Source: CAD feature listing. Evaluate the final solid. Frame: model axes, mm. Face numbers are marked on the shaded views. A direction names the side the tool comes from. Give positions to 0.01 mm unless a question says otherwise; leave off trailing zeros. Loops run counter-clockwise (first coordinate to the right, second up) from the corner with the lowest first, then second, coordinate; pieces in that order, holes last. Notation, with made-up numbers: (54.5, -34) -> (93.5, -34) arc R16 cw to (93.5, -23) -> close; hole circle Ø8 at (5.5, -2). An arc over 180 degrees is marked (long way). Return JSON: item names as keys, results as strings. Group by question number.
```python
from build123d import *

# Parameters (mm, degrees)
SKETCH2_W            = 230
SKETCH2_H            = 40
BOSS_EXTRUDE1_DEPTH  = 80
SKETCH3_W            = 200.4
SKETCH3_H            = 10
CUT_EXTRUDE1_DEPTH   = 30
SKETCH6_R            = 25
BOSS_EXTRUDE3_DEPTH  = 50
SKETCH7_R            = 12.5
CUT_EXTRUDE2_DEPTH   = 50
SKETCH8_R            = 26.5
CUT_EXTRUDE3_DEPTH   = 25
CUT_EXTRUDE4_START   = 40
SKETCH11_R           = 26.5
CUT_EXTRUDE4_DEPTH   = 40
SKETCH14_W           = 12.614661349
SKETCH14_H           = 40
CUT_EXTRUDE6_DEPTH   = 50
FILLET3_R            = 20
FILLET3_OF_MIRROR5_R = 20
FILLET3_OF_MIRROR8_R = 20
SKETCH15_R           = 27.771194789
CUT_EXTRUDE7_DEPTH   = 5
SKETCH21_R           = 27.635802496
CUT_EXTRUDE8_DEPTH   = 5


with BuildPart() as part:
    # Sketch2 → Boss-Extrude1 (new body)
    with BuildSketch(Plane.XY):
        with Locations((115, 20)):
            Rectangle(SKETCH2_W, SKETCH2_H)
    extrude(amount=BOSS_EXTRUDE1_DEPTH)

    # Sketch3 → Cut-Extrude1 (cut)
    with BuildSketch(Plane.XY.offset(80)):
        with Locations((115, 20)):
            Rectangle(SKETCH3_W, SKETCH3_H)
    extrude(amount=-CUT_EXTRUDE1_DEPTH, mode=Mode.SUBTRACT)

    # Sketch6 → Boss-Extrude3 (add)
    with BuildSketch(Plane(origin=(140, 0, 0), x_dir=(0, 0, -1), z_dir=(1, 0, 0))):
        with Locations((10, 20)):
            Circle(SKETCH6_R)
    boss_extrude3 = extrude(amount=BOSS_EXTRUDE3_DEPTH)

    # Sketch7 → Cut-Extrude2 (cut)
    with BuildSketch(Plane.ZY.offset(-140)):
        with Locations(Location((-10, 20, 0), (0, 0, 36.869897646))):
            Circle(SKETCH7_R)
    cut_extrude2 = extrude(amount=-CUT_EXTRUDE2_DEPTH, mode=Mode.SUBTRACT)

    # Sketch8 → Cut-Extrude3 (cut)
    with BuildSketch(Plane.ZY.offset(-140)):
        with Locations((-10, 20)):
            Circle(SKETCH8_R)
    cut_extrude3 = extrude(amount=CUT_EXTRUDE3_DEPTH, mode=Mode.SUBTRACT)

    # Sketch11 → Cut-Extrude4 (cut)
    with BuildSketch(Plane(origin=(190, 0, 0), x_dir=(0, 0, -1), z_dir=(1, 0, 0)).offset(CUT_EXTRUDE4_START)):
        with Locations((10, 20)):
            Circle(SKETCH11_R)
    cut_extrude4 = extrude(amount=-CUT_EXTRUDE4_DEPTH, mode=Mode.SUBTRACT)

    # Mirror1: Boss-Extrude3, Cut-Extrude2, Cut-Extrude3, Cut-Extrude4 across plane
    add(boss_extrude3.mirror(Plane(origin=(115, 0, 0), x_dir=(0, 0, 1), z_dir=(1, 0, 0))))
    add(cut_extrude2.mirror(Plane(origin=(115, 0, 0), x_dir=(0, 0, 1), z_dir=(1, 0, 0))), mode=Mode.SUBTRACT)
    add(cut_extrude3.mirror(Plane(origin=(115, 0, 0), x_dir=(0, 0, 1), z_dir=(1, 0, 0))), mode=Mode.SUBTRACT)
    add(cut_extrude4.mirror(Plane(origin=(115, 0, 0), x_dir=(0, 0, 1), z_dir=(1, 0, 0))), mode=Mode.SUBTRACT)

    # Sketch14 → Cut-Extrude6 (cut)
    with BuildSketch(Plane(origin=(90, 0, 0), x_dir=(0, 0, -1), z_dir=(1, 0, 0))):
        with Locations((-13.692669326, 20)):
            Rectangle(SKETCH14_W, SKETCH14_H)
    cut_extrude6 = extrude(amount=CUT_EXTRUDE6_DEPTH, mode=Mode.SUBTRACT)

    # Fillet3
    fillet3_edges = [part.edges().sort_by_distance(p)[0] for p in [
        (115, 40, 20),
        (115, 0, 20),
    ]]
    fillet(fillet3_edges, radius=FILLET3_R - 0.0001)  # a hair under: the kernel refuses the full size

    # Mirror5: Cut-Extrude6 across plane
    add(cut_extrude6.mirror(Plane.ZY.offset(-165)), mode=Mode.SUBTRACT)

    # Fillet3 of Mirror5
    fillet3_of_mirror5_edges = [part.edges().sort_by_distance(p)[0] for p in [
        (210, 40, 20),
        (210, 0, 20),
    ]]
    fillet(fillet3_of_mirror5_edges, radius=FILLET3_OF_MIRROR5_R - 0.0001)  # a hair under: the kernel refuses the full size

    # Mirror8: Cut-Extrude6 across plane
    add(cut_extrude6.mirror(Plane(origin=(65, 0, 0), x_dir=(0, 0, 1), z_dir=(1, 0, 0))), mode=Mode.SUBTRACT)

    # Fillet3 of Mirror8
    fillet3_of_mirror8_edges = [part.edges().sort_by_distance(p)[0] for p in [
        (20, 40, 20),
        (20, 0, 20),
    ]]
    fillet(fillet3_of_mirror8_edges, radius=FILLET3_OF_MIRROR8_R - 0.0001)  # a hair under: the kernel refuses the full size

    # Sketch15 → Cut-Extrude7 (cut)
    with BuildSketch(Plane(origin=(90, 0, 0), x_dir=(0, 0, -1), z_dir=(1, 0, 0))):
        with Locations((10, 20)):
            Circle(SKETCH15_R)
    extrude(amount=-CUT_EXTRUDE7_DEPTH, mode=Mode.SUBTRACT)

    # Sketch21 → Cut-Extrude8 (cut)
    with BuildSketch(Plane.ZY.offset(-140)):
        with Locations((-10.3298846, 20.067055547)):
            Circle(SKETCH21_R)
    extrude(amount=-CUT_EXTRUDE8_DEPTH, mode=Mode.SUBTRACT)


solid = part.part
```
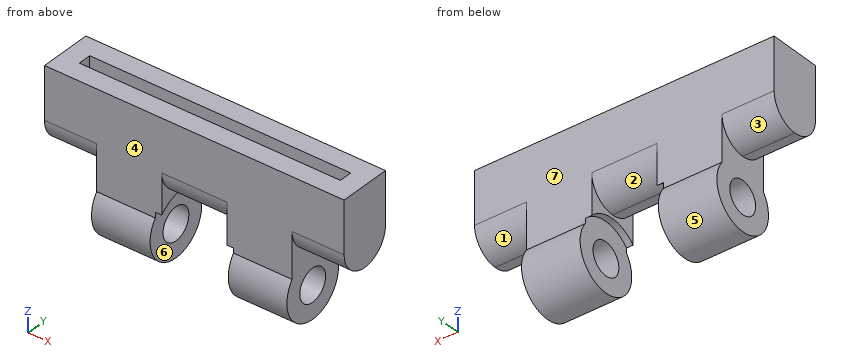
1) Cut plane C-C on x = 58.5. Return loops of the section in (y, z).
2) Reachability of the marked faces 1, 2, 3 and 4 from +Z, -Z, +X, -X, +Y, -Y: full face, straight path, thin tool, end or side. Return the list, or none.
3) Mould query, pull axis Y, two halves, no side actions, for the marked faces 5, 6 and 7. Classes: released by +Y, released by -Y, zero draft, split by the parting line, or undercut.
4) Cut plane A-A on z = 55. Return loops of the section in (x, y), then the cut area to 3 significant figures.
5) Contact query for flat-ended pins moving along their axis: P1, Ø15, axis at x = 117, z = 66.5, coming from the +Y side; P2, Ø8, axis at y = 19.5, z = 58, coming from the -X side; P3, Ø12, axis at y = 32, z = -7, coming from the -X side; P4, Ø10, axis at x = 27.5, y = 34.5, coming from the -Z side. Output: stop coordinate, or through.
6) Cut plane B-B on z = -10. Return loops of the section in (x, y).
7) Material intervals for line 1 (Y direction, x = 49, z = -10); line 2 (X direction, y = 15, z = 14); line 3 (Z direction, x = 156, y = 20), sorted ascending.
Calculated:
{
 "1": {"outline": "(0, 5) arc R25 ccw (long way) to (40, 5) -> (40, 80) -> (25, 80) -> (25, 50) -> (15, 50) -> (15, 80) -> (0, 80) -> close; hole circle Ø25 at (20, -10)"},
 "2": {"face 1": "-Z, +X, +Y", "face 2": "-Z, +Y", "face 3": "-Z, -X, +Y", "face 4": "+Z, +X, -X, -Y"},
 "3": {"face 5": "split by the parting line", "face 6": "undercut", "face 7": "released by +Y"},
 "4": {"outline": "(0, 0) -> (230, 0) -> (230, 40) -> (0, 40) -> close; hole (14.8, 15) -> (215.2, 15) -> (215.2, 25) -> (14.8, 25) -> close", "area": "7,200 mm2"},
 "5": {"P1": "y = 40", "P2": "x = 0", "P3": "x = 40", "P4": "z = 22.4"},
 "6": {"outline": "(40, -5) -> (85, -5) -> (85, 7.5) -> (40, 7.5) -> close; (40, 32.5) -> (85, 32.5) -> (85, 45) -> (40, 45) -> close; (145, -5) -> (190, -5) -> (190, 7.5) -> (145, 7.5) -> close; (145, 32.5) -> (190, 32.5) -> (190, 45) -> (145, 45) -> close"},
 "7": {"line 1": "-5 to 7.5, 32.5 to 45", "line 2": "40 to 85, 145 to 190", "line 3": "-35 to -22.5, 2.5 to 50"}
}
